from build123d import *

# Parameters (mm, degrees)
CROQUIS1_W                 = 39.618473901
CROQUIS1_H                 = 62.206373563
SALIENTE_EXTRUIR1_DEPTH    = 3
CROQUIS2_R                 = 10
SALIENTE_EXTRUIR2_DEPTH    = 15
CROQUIS3_R                 = 4
CORTAR_EXTRUIR1_DEPTH      = 63.693025162
CORTAR_EXTRUIR3_DEPTH      = 63.693025162
CORTAR_EXTRUIR3_DEPTH_BACK = 63.693025162
CROQUIS5_R                 = 2
CROQUIS6_R                 = 3
CORTAR_EXTRUIR4_DEPTH      = 10
CORTAR_EXTRUIR5_DEPTH      = 63.69302519
CORTAR_EXTRUIR5_DEPTH_BACK = 63.69302519
CROQUIS7_R                 = 2


with BuildPart() as part:
    # Croquis1 → Saliente-Extruir1 (new body)
    with BuildSketch(Plane.XY):
        with Locations((28.835278497, -4.112243371)):
            Rectangle(CROQUIS1_W, CROQUIS1_H)
    extrude(amount=SALIENTE_EXTRUIR1_DEPTH)

    # Croquis2 → Saliente-Extruir2 (add)
    with BuildSketch(Plane.XY.offset(3)):
        with Locations((28.835278496, -4.112243372)):
            Circle(CROQUIS2_R)
    extrude(amount=SALIENTE_EXTRUIR2_DEPTH)

    # Croquis3 → Cortar-Extruir1 (cut, through all)
    with BuildSketch(Plane.XY.offset(18)):
        with Locations((28.835278496, -4.112243372)):
            Circle(CROQUIS3_R)
    extrude(amount=-CORTAR_EXTRUIR1_DEPTH, mode=Mode.SUBTRACT)

    # Croquis5 → Cortar-Extruir3 (cut, two sides: drawn at the far end of the back side and taken through both)
    with BuildSketch(Plane(origin=(0, 0, 0), x_dir=(0, 0, -1), z_dir=(1, 0, 0)).offset(-CORTAR_EXTRUIR3_DEPTH_BACK)):
        with Locations(Location((-7.893110832, -4.112243372, 0), (0, 0, 180))):
            Circle(CROQUIS5_R)
    extrude(amount=CORTAR_EXTRUIR3_DEPTH + CORTAR_EXTRUIR3_DEPTH_BACK, mode=Mode.SUBTRACT)

    # Croquis6 → Cortar-Extruir4 (cut)
    with BuildSketch(Plane(origin=(0, 0, 0), x_dir=(-1, 0, 0), z_dir=(0, 0, -1))):
        with Locations((-40.490083912, -29.215430153)):
            Circle(CROQUIS6_R)
        with Locations((-28.490083912, -29.215430153)):
            Circle(CROQUIS6_R)
        with Locations((-16.490083912, -29.215430153)):
            Circle(CROQUIS6_R)
        with Locations((-28.490083912, 20.99094341)):
            Circle(CROQUIS6_R)
        with Locations((-40.490083912, 20.99094341)):
            Circle(CROQUIS6_R)
        with Locations((-16.490083912, 20.99094341)):
            Circle(CROQUIS6_R)
    extrude(amount=-CORTAR_EXTRUIR4_DEPTH, mode=Mode.SUBTRACT)

    # Croquis7 → Cortar-Extruir5 (cut, two sides: drawn at the far end of the back side and taken through both)
    with BuildSketch(Plane(origin=(0, 0, 0), x_dir=(1, 0, 0), z_dir=(0, 1, 0)).offset(-CORTAR_EXTRUIR5_DEPTH_BACK)):
        with Locations(Location((28.835278496, -13.615803353, 0), (0, 0, 270))):
            Circle(CROQUIS7_R)
    extrude(amount=CORTAR_EXTRUIR5_DEPTH + CORTAR_EXTRUIR5_DEPTH_BACK, mode=Mode.SUBTRACT)


solid = part.part
Geometry check sheet. Reference: the model listing, model coordinates, mm. A direction names the side the tool comes from. Round coordinates to 2 decimals unless told otherwise and drop trailing zeros. Write each loop counter-clockwise with the first axis right and the second up, starting at its lowest first coordinate (ties: lowest second). Pieces come first, ordered by that corner, then holes. Notation, with made-up numbers: (-2.5, 59.25) -> (54.5, 59.25) arc R30 ccw to (54.5, 92.25) -> close; hole circle Ø7 at (6, 41.25). An arc over 180 degrees is marked (long way). One line per item, written item: value. Start each with the question number.
(1) Cross-section at D-D, the plane z = 1.25. Record the cut outline in (x, y).
(2) Cross-section at B-B, the plane y = 2. Record the cut outline in (x, z).
(3) Access from +Z, -Z, +X, -X, +Y, -Y to the whole of each face (thin tool, end or side, straight path). Record for faces 1 (the cylindrical face through (19.487, -29.084, 1.479)), 2 (the cylindrical face through (38.073, -7.942, 10.395)).
(4) Cross-section at C-C, the plane x = 17.5. Record the cut outline in (y, z), and give its area (3 significant figures).
(5) Go/stop test with flat-tipped pins: pin 1 Ø4 at (y, z) = (4, 14) entering from -X; pin 2 Ø6.5 at (x, z) = (28.84, 13.62) entering from +Y; pin 3 Ø2 at (x, y) = (23, -18) entering from +Z. Record where each tip stops, or that it passes through.
(6) Draft check along Z on faces 3 (the cylindrical face through (30.82, 2.58, 13.36)), 4 (the cylindrical face through (31.487, 21.123, 1.479)), 5 (the flat face through (33, -4, 0)), 6 (the flat face through (28.7, -8.4, 18)). Enter one of: +Z half, -Z half, draft (parallel to the pull), parting line (faces both ways), or undercut.
(7) Scan lines: line 1 (X direction, y = -29, z = 2.75); line 2 (Y direction, x = 34.5, z = 6.5); line 3 (X direction, y = 23.5, z = 2). Record each from-to range of solid material in increasing order. Write a range as [from, to].
(8) Cross-section at A-A, the plane z = 7.5. Record the cut outline in (x, y), and give its area (3 significant figures).
Answer:
1. outline: (9.03, -35.22) -> (48.64, -35.22) -> (48.64, 26.99) -> (9.03, 26.99) -> close; hole circle Ø6 at (16.49, -29.22); hole circle Ø6 at (16.49, 20.99); hole circle Ø8 at (28.84, -4.11); hole circle Ø6 at (28.49, -29.22); hole circle Ø6 at (28.49, 20.99); hole circle Ø6 at (40.49, -29.22); hole circle Ø6 at (40.49, 20.99)
2. outline: (9.03, 0) -> (48.64, 0) -> (48.64, 3) -> (36.75, 3) -> (36.75, 18) -> (20.92, 18) -> (20.92, 3) -> (9.03, 3) -> close; hole circle Ø4 at (28.84, 13.62)
3. face 1: +Z, -Z
3. face 2: +Z
4. outline: (-35.22, 0) -> (-32.04, 0) -> (-32.04, 3) -> (-35.22, 3) -> close; (-26.39, 0) -> (18.17, 0) -> (18.17, 3) -> (-26.39, 3) -> close; (23.82, 0) -> (26.99, 0) -> (26.99, 3) -> (23.82, 3) -> close
4. area: 153 mm²
5. pin 1: x = 20.92
5. pin 2: y = 5.89
5. pin 3: z = 3
6. face 3: undercut
6. face 4: draft
6. face 5: -Z half
6. face 6: +Z half
7. line 1: [9.03, 13.5], [19.48, 25.5], [31.48, 37.5], [43.48, 48.64]
7. line 2: [-12.35, -5.55], [-2.68, 4.13]
7. line 3: [9.03, 14.85], [18.13, 26.85], [30.13, 38.85], [42.13, 48.64]
8. outline: (19.03, -6.07) arc R10 ccw to (38.64, -6.07) -> (32.32, -6.07) arc R4 cw to (25.35, -6.07) -> close; (19.03, -2.15) -> (25.35, -2.15) arc R4 cw to (32.32, -2.15) -> (38.64, -2.15) arc R10 ccw to start
8. area: 216 mm²
